Could you check a few things on this model? Use its own coordinates, in mm. Coordinates: 2 decimals unless noted, no trailing zeros. Loops run counter-clockwise (first coordinate to the right, second up) from the corner with the lowest first, then second, coordinate; pieces in that order, holes last.
from build123d import *

# Parameters (mm, degrees)
BOSS_EXTRUDE1_DEPTH = 10


with BuildPart() as part:
    # Sketch1 → Boss-Extrude1 (new body)
    with BuildSketch(Plane.XY):
        with BuildLine():
            Line((-96.875667103, 70.38429208), (-107.329159547, 38.211750479))
            ThreePointArc((-107.329159547, 38.211750479), (-111.329892944, 36.173274997), (-109.291417462, 32.172541601))
            Line((-109.291417462, 32.172541601), (-119.744909905, 0))
            Line((-119.744909905, 0), (-161.803398875, 0))
            Line((-161.803398875, 0), (-130.901699437, 95.10565163))
            Line((-130.901699437, 95.10565163), (-50, 153.884176859))
            Line((-50, 153.884176859), (50, 153.884176859))
            Line((50, 153.884176859), (130.901699437, 95.10565163))
            Line((130.901699437, 95.10565163), (161.803398875, 0))
            Line((161.803398875, 0), (119.744909905, 0))
            Line((119.744909905, 0), (109.291417462, 32.172541601))
            ThreePointArc((109.291417462, 32.172541601), (111.329892944, 36.173274997), (107.329159547, 38.211750479))
            Line((107.329159547, 38.211750479), (96.875667103, 70.38429208))
            Line((96.875667103, 70.38429208), (69.508068584, 90.268016293))
            ThreePointArc((69.508068584, 90.268016293), (68.805657803, 94.702863426), (64.37081067, 94.000452645))
            Line((64.37081067, 94.000452645), (37.003212151, 113.884176859))
            Line((37.003212151, 113.884176859), (3.175, 113.884176859))
            ThreePointArc((3.175, 113.884176859), (0, 117.059176859), (-3.175, 113.884176859))
            Line((-3.175, 113.884176859), (-37.003212151, 113.884176859))
            Line((-37.003212151, 113.884176859), (-64.37081067, 94.000452645))
            ThreePointArc((-64.37081067, 94.000452645), (-68.805657803, 94.702863426), (-69.508068584, 90.268016293))
            Line((-69.508068584, 90.268016293), (-96.875667103, 70.38429208))
        make_face()
    extrude(amount=BOSS_EXTRUDE1_DEPTH)


solid = part.part
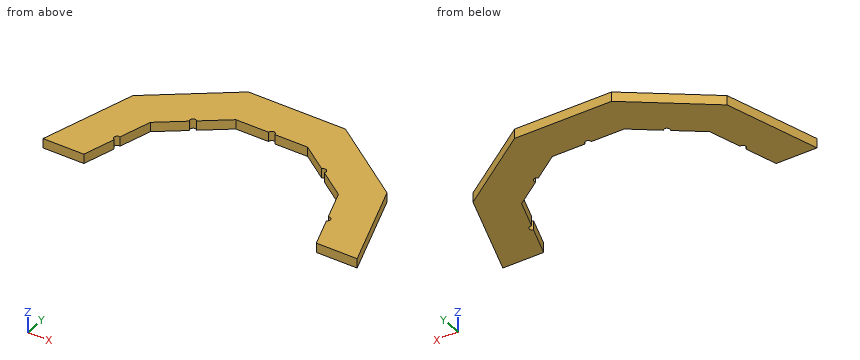
(1) Imagine slicing it at B-B, the plane z = 7.5. Write out the boundary of the cut face in (x, y) (3 decimals), and give its area (3 significant figures).
Answers:
outline: (-161.803, 0) - (-119.745, 0) - (-109.291, 32.173) arc R3.175 cw to (-107.329, 38.212) - (-96.876, 70.384) - (-69.508, 90.268) arc R3.175 cw to (-64.371, 94) - (-37.003, 113.884) - (-3.175, 113.884) arc R3.175 cw to (3.175, 113.884) - (37.003, 113.884) - (64.371, 94) arc R3.175 cw to (69.508, 90.268) - (96.876, 70.384) - (107.329, 38.212) arc R3.175 cw to (109.291, 32.173) - (119.745, 0) - (161.803, 0) - (130.902, 95.106) - (50, 153.884) - (-50, 153.884) - (-130.902, 95.106) - close
area: 17,300 mm2
(2) I need wall thicknesses on probe 1 along Y at (x, z) = (-35.5, 6); probe 2 along X at (y, z) = (60.5, 4.25); probe 3 along X at (y, z) = (84, 5.25). Which ranges of each line are inside material? Lowest first, please.
Answers:
probe 1: y = 113.88 to 153.88
probe 2: x = -142.15 to -100.09, 100.09 to 142.15
probe 3: x = -134.51 to -78.14, 78.14 to 134.51
(3) Imagine slicing it at D-D, the plane y = 74. Write out the boundary of the cut face in (x, z), and give its area (3 significant figures).
Answers:
outline: (-137.76, 0) - (-91.9, 0) - (-91.9, 10) - (-137.76, 10) - close; (91.9, 0) - (137.76, 0) - (137.76, 10) - (91.9, 10) - close
area: 917 mm2
(4) For pin 1 (5 mm diameter, centred on x = -64.5, z = 6.5, fed in from +Y); pin 2 (5 mm diameter, centred on y = 49.5, z = 7.5, fed in from +X); pin 3 (1.5 mm diameter, centred on x = -64, z = 8, fed in from +Y), each with a flat end and sliding along its axis, tell me the tip position at first contact or that it passes through.
Answers:
pin 1: stops at y = 145.17
pin 2: stops at x = 146.53
pin 3: stops at y = 144.26
(5) Imagine slicing it at C-C, the plane x = 0. Write out the boundary of the cut face in (y, z), and give its area (3 significant figures).
Answers:
outline: (117.06, 0) - (153.88, 0) - (153.88, 10) - (117.06, 10) - close
area: 368 mm2
(6) Imagine slicing it at A-A, the plane y = 43. Write out the boundary of the cut face in (x, z).
Answers:
outline: (-147.83, 0) - (-105.77, 0) - (-105.77, 10) - (-147.83, 10) - close; (105.77, 0) - (147.83, 0) - (147.83, 10) - (105.77, 10) - close
